from build123d import *

# Parameters (mm, degrees)
SKETCH1_R           = 2.159
SKETCH1_R_2         = 16.51
BOSS_EXTRUDE1_DEPTH = 1.524
SKETCH2_R           = 2.159
SKETCH2_R_2         = 13.335
BOSS_EXTRUDE2_DEPTH = 2
FILLET1_R           = 2.54


with BuildPart() as part:
    # Sketch1 → Boss-Extrude1 (new body)
    with BuildSketch(Plane.XY):
        with BuildLine():
            ThreePointArc((15.272530034, -14.716368688), (21.117163446, -12.192), (20.381014152, -5.868214645))
            ThreePointArc((20.381014152, -5.868214645), (18.367532789, 10.6045), (5.108484119, 20.584583333))
            ThreePointArc((5.108484119, 20.584583333), (0, 24.384), (-5.108484119, 20.584583333))
            ThreePointArc((-5.108484119, 20.584583333), (-18.367532789, 10.6045), (-20.381014152, -5.868214645))
            ThreePointArc((-20.381014152, -5.868214645), (-21.117163446, -12.192), (-15.272530034, -14.716368688))
            ThreePointArc((-15.272530034, -14.716368688), (0, -21.209), (15.272530034, -14.716368688))
        make_face()
        with Locations((0, 19.05)):
            Circle(SKETCH1_R, mode=Mode.SUBTRACT)
        with Locations((16.497783942, -9.525)):
            Circle(SKETCH1_R, mode=Mode.SUBTRACT)
        with Locations((-16.497783942, -9.525)):
            Circle(SKETCH1_R, mode=Mode.SUBTRACT)
        Circle(SKETCH1_R_2, mode=Mode.SUBTRACT)
    extrude(amount=BOSS_EXTRUDE1_DEPTH)

    # Sketch2 → Boss-Extrude2 (add)
    with BuildSketch(Plane.XY):
        with BuildLine():
            ThreePointArc((-20.381014152, -5.868214645), (-21.117163446, -12.192), (-15.272530034, -14.716368688))
            ThreePointArc((-15.272530034, -14.716368688), (0, -21.209), (15.272530034, -14.716368688))
            ThreePointArc((15.272530034, -14.716368688), (21.117163446, -12.192), (20.381014152, -5.868214645))
            ThreePointArc((20.381014152, -5.868214645), (18.367532789, 10.6045), (5.108484119, 20.584583333))
            ThreePointArc((5.108484119, 20.584583333), (0, 24.384), (-5.108484119, 20.584583333))
            ThreePointArc((-5.108484119, 20.584583333), (-18.367532789, 10.6045), (-20.381014152, -5.868214645))
        make_face()
        with Locations((0, 19.05)):
            Circle(SKETCH2_R, mode=Mode.SUBTRACT)
        with Locations((-16.497783942, -9.525)):
            Circle(SKETCH2_R, mode=Mode.SUBTRACT)
        Circle(SKETCH2_R_2, mode=Mode.SUBTRACT)
        with Locations((16.497783942, -9.525)):
            Circle(SKETCH2_R, mode=Mode.SUBTRACT)
    extrude(amount=-BOSS_EXTRUDE2_DEPTH)

    # Fillet1
    fillet1_edges = [part.edges().sort_by_distance(p)[0] for p in [
        (15.272530034, -14.716368688, -0.238),
        (-15.272530034, -14.716368688, -0.238),
        (-20.381014152, -5.868214645, -0.238),
        (-5.108484119, 20.584583333, -0.238),
        (5.108484119, 20.584583333, -0.238),
        (20.381014152, -5.868214645, -0.238),
    ]]
    fillet(fillet1_edges, radius=FILLET1_R)


solid = part.part
Read the model definition and answer for the solid it produces. Units are mm, in the model's axes. A direction names the side the tool comes from. Round coordinates to 2 decimals unless told otherwise and drop trailing zeros. Write each loop counter-clockwise with the first axis right and the second up, starting at its lowest first coordinate (ties: lowest second). Pieces come first, ordered by that corner, then holes. Notation, with made-up numbers: (35.25, -22) - (82.25, -22) arc R24 ccw to (82.25, 6) - close; hole circle Ø4 at (53, -26.75). An arc over 180 degrees is marked (long way). Use a Markdown table: item, result.
(1) The part is cut by section B-B (y = 0). Write down the section's boundary in (x, z) (3 decimals).
Reported:
| item | result |
|---|---|
| outline | (-21.209, -2) - (-13.335, -2) - (-13.335, 0) - (-16.51, 0) - (-16.51, 1.524) - (-21.209, 1.524) - close; (13.335, -2) - (21.209, -2) - (21.209, 1.524) - (16.51, 1.524) - (16.51, 0) - (13.335, 0) - close |
(2) The mould has two halves that part along Y. Classify faces 1 (the cylindrical face through (0.081, 24.383, -0.213)), 2 (the flat face through (1, 14, 0)), 3 (the cylindrical face through (-0.222, -21.208, -0.213)): released by +Y, released by -Y, zero draft, split by the parting line, or undercut.
Reported:
| item | result |
|---|---|
| face 1 | released by +Y |
| face 2 | undercut |
| face 3 | released by -Y |
(3) The part is cut by section C-C (x = -8). Write down the section's boundary in (y, z), then the cut area to 3 significant figures.
Reported:
| item | result |
|---|---|
| outline | (-19.64, -2) - (-10.67, -2) - (-10.67, 0) - (-14.44, 0) - (-14.44, 1.52) - (-19.64, 1.52) - close; (10.67, -2) - (19.64, -2) - (19.64, 1.52) - (14.44, 1.52) - (14.44, 0) - (10.67, 0) - close |
| area | 51.7 mm2 |
(4) The part is cut by section A-A (x = 0). Write down the section's boundary in (y, z) (3 decimals), then the cut area to 3 significant figures.
Reported:
| item | result |
|---|---|
| outline | (-21.209, -2) - (-13.335, -2) - (-13.335, 0) - (-16.51, 0) - (-16.51, 1.524) - (-21.209, 1.524) - close; (13.335, -2) - (16.891, -2) - (16.891, 1.524) - (16.51, 1.524) - (16.51, 0) - (13.335, 0) - close; (21.209, -2) - (24.384, -2) - (24.384, 1.524) - (21.209, 1.524) - close |
| area | 41.8 mm2 |
(5) Which of the six approach directions +Z, -Z, +X, -X, +Y, -Y give full straight-line access (tool end or side, diameter ignored) to faces 4 (the cylindrical face through (15.748, 4.959, 0.751)), 5 (the cylindrical face through (-1.74, 13.22, -0.99))?
Reported:
| item | result |
|---|---|
| face 4 | +Z |
| face 5 | +Z, -Z |
(6) Straight lines are drawn through the part: line 1 along Y through (x, z) = (0, 1.3); line 2 along X through (y, z) = (-8, -1.8); line 3 along Y through (x, z) = (-11, 1.3). For each, find the intervals that lie inside material, in ascending order. Write a range as [from, to].
Reported:
| item | result |
|---|---|
| line 1 | [-21.21, -16.51], [16.51, 16.89], [21.21, 24.38] |
| line 2 | [-21.61, -18.03], [-14.97, -10.67], [10.67, 14.97], [18.03, 21.61] |
| line 3 | [-18.13, -12.31], [12.31, 18.13] |
(7) The part is cut by section D-D (y = 19.05). Write down the section's boundary in (x, z).
Reported:
| item | result |
|---|---|
| outline | (-9.32, -2) - (-2.16, -2) - (-2.16, 1.52) - (-9.32, 1.52) - close; (2.16, -2) - (9.32, -2) - (9.32, 1.52) - (2.16, 1.52) - close |
